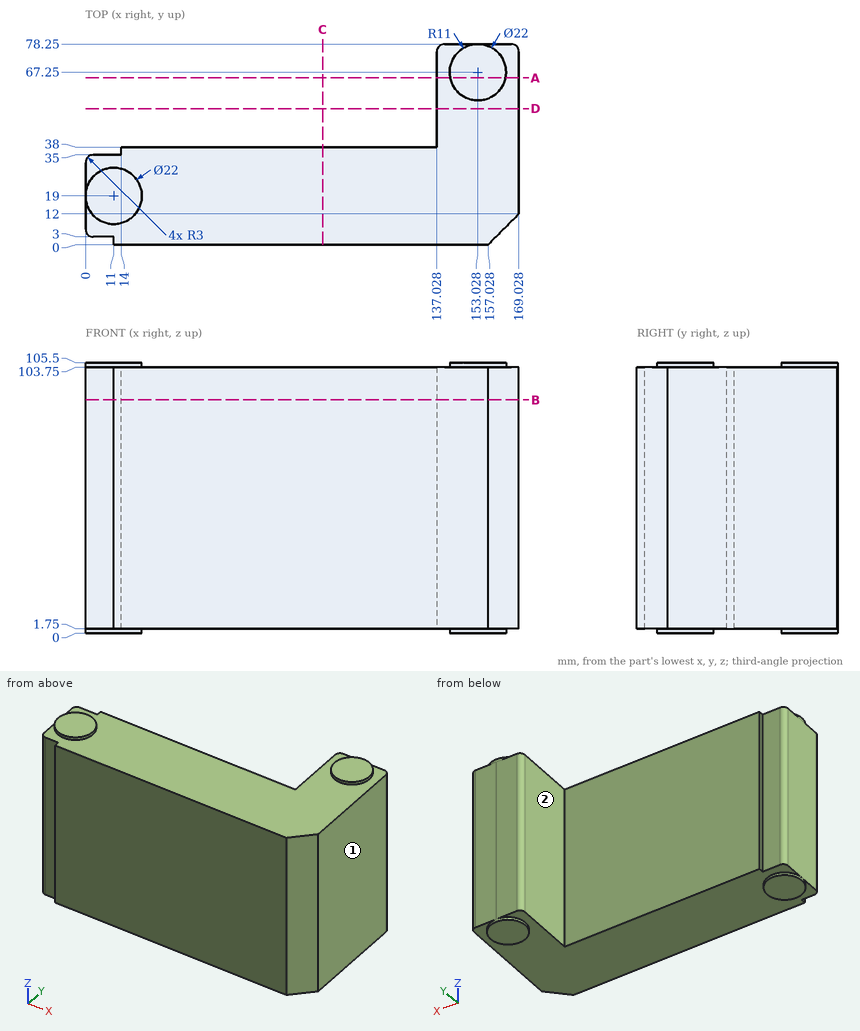
Study the drawing (mm; zero at the part's minimum x, y, z) and answer. A direction names the side the tool comes from. Give positions to 0.01 mm unless a question says otherwise; leave off trailing zeros. Loops run counter-clockwise (first coordinate to the right, second up) from the corner with the lowest first, then second, coordinate; pieces in that order, holes last. Notation, with made-up numbers: (-7.75, -27.75) - (21.25, -27.75) arc R22 ccw to (21.25, -18.75) - close; hole circle Ø3 at (-3.5, 41.25). An arc over 180 degrees is marked (long way). Answer in a Markdown table with one row per item. Add a question column.
Q1. Each of these flat-tipped pins is pushed along its axis until it touches: P1, Ø3.5, axis at y = 36, z = 56.5, coming from the -X side (1 decimal); P2, Ø6, axis at y = 52, z = 92, coming from the -X side; P3, Ø2.5, axis at x = 8.5, z = 37.5, coming from the -Y side. Where does it stop, or does it pass through?
Q2. The part is cut by section C-C (x = 92.5). Determine the outline of the cut face in (y, z), and give its area (3 significant figures).
Q3. The part is cut by section D-D (y = 53). Determine the outline of the cut face in (x, z).
Q4. Consider line 1 along X through (y, z) = (58.5, 69.5); line 2 along Z through (x, y) = (105, 4.5); line 3 along Y through (x, z) = (32.5, 68.5). Determine where each line is inside the solid, lowest interval first.
Q5. The part is cut by section B-B (z = 91). Determine the outline of the cut face in (x, y).
Q6. The part is cut by section A-A (y = 65). Determine the outline of the cut face in (x, z).
Q7. A tool of negligible diameter and unlimited length cuts with its end or side. For the marked faces 1 and 2, from which of +Z, -Z, +X, -X, +Y, -Y can it reach the whole face along a straight path? Write none if from no direction.
Solution:
| question | item | result |
|---|---|---|
| 1 | P1 | stops at x = 1 |
| 1 | P2 | stops at x = 137.03 |
| 1 | P3 | stops at y = 3 |
| 2 | outline | (0, 1.75) - (38, 1.75) - (38, 103.75) - (0, 103.75) - close |
| 2 | area | 3,880 mm² |
| 3 | outline | (137.03, 1.75) - (169.03, 1.75) - (169.03, 103.75) - (137.03, 103.75) - close |
| 4 | line 1 | x = 137.03 to 169.03 |
| 4 | line 2 | z = 1.75 to 103.75 |
| 4 | line 3 | y = 0 to 38 |
| 5 | outline | (0, 6) arc R3 ccw to (3, 3) - (11, 3) - (11, 0) - (157.03, 0) - (169.03, 12) - (169.03, 75.25) arc R3 ccw to (166.03, 78.25) - (153.09, 78.25) arc R11 ccw to (152.97, 78.25) - (140.03, 78.25) arc R3 ccw to (137.03, 75.25) - (137.03, 38) - (14, 38) - (14, 35) - (3, 35) arc R3 ccw to (0, 32) - close |
| 6 | outline | (137.03, 1.75) - (142.26, 1.75) - (142.26, 0) - (163.8, 0) - (163.8, 1.75) - (169.03, 1.75) - (169.03, 103.75) - (163.8, 103.75) - (163.8, 105.5) - (142.26, 105.5) - (142.26, 103.75) - (137.03, 103.75) - close |
| 7 | face 1 | +Z, -Z, +X, +Y, -Y |
| 7 | face 2 | +Z, -Z, -X, +Y |
